from build123d import *

# Parameters (mm, degrees)
BODYSKETCH_R = 0.5969
BODY_DEPTH   = 0.889


with BuildPart() as part:
    # BodySketch → Body (new body)
    with BuildSketch(Plane.XY):
        with BuildLine():
            Line((0.152065789, -5.941654396), (0.22225, -8.683956424))
            ThreePointArc((0.22225, -8.683956424), (1.368573357, -8.578315756), (2.490862191, -8.322024981))
            ThreePointArc((2.490862191, -8.322024981), (2.671680086, -8.204051371), (2.759354342, -8.006754365))
            Line((2.759354342, -8.006754365), (2.871664527, -7.153673811))
            ThreePointArc((2.871664527, -7.153673811), (3.142109784, -6.428451286), (3.702191114, -5.894225443))
            ThreePointArc((3.702191114, -5.894225443), (0, 7.5946), (-3.702191114, -5.894225443))
            ThreePointArc((-3.702191114, -5.894225443), (-3.142109784, -6.428451286), (-2.871664527, -7.153673811))
            Line((-2.871664527, -7.153673811), (-2.759354342, -8.006754365))
            ThreePointArc((-2.759354342, -8.006754365), (-2.671680086, -8.204051371), (-2.490862191, -8.322024981))
            ThreePointArc((-2.490862191, -8.322024981), (-1.368573357, -8.578315756), (-0.22225, -8.683956424))
            Line((-0.22225, -8.683956424), (-0.152065789, -5.941654396))
            ThreePointArc((-0.152065789, -5.941654396), (0, 5.9436), (0.152065789, -5.941654396))
        make_face()
        with Locations((1.0414, -7.445926712)):
            Circle(BODYSKETCH_R, mode=Mode.SUBTRACT)
        with Locations((-1.0414, -7.445926712)):
            Circle(BODYSKETCH_R, mode=Mode.SUBTRACT)
    extrude(amount=BODY_DEPTH)


solid = part.part
For this review, take the finished solid that the model builds, in its own axes (mm). Round coordinates to 2 decimals unless told otherwise and drop trailing zeros. Loops run counter-clockwise (first coordinate to the right, second up) from the corner with the lowest first, then second, coordinate; pieces in that order, holes last. Notation, with made-up numbers: (39, -2.75) - (98, -2.75) arc R30 cw to (98, 31.25) - close; hole circle Ø6 at (-4.5, -16.5). An arc over 180 degrees is marked (long way). One line per question, with ' | ' between items.
Q1. Take a section at B-B (z = 0.4). Give the boundary of the cut face in (x, y), and give its area (3 significant figures).
Taken from the geometry:
outline: (-3.7, -5.89) arc R1.73 cw to (-2.87, -7.15) - (-2.76, -8.01) arc R0.38 ccw to (-2.49, -8.32) arc R8.69 ccw to (-0.22, -8.68) - (-0.15, -5.94) arc R5.94 cw (long way) to (0.15, -5.94) - (0.22, -8.68) arc R8.69 ccw to (2.49, -8.32) arc R0.38 ccw to (2.76, -8.01) - (2.87, -7.15) arc R1.73 cw to (3.7, -5.89) arc R7.25 ccw (long way) to start; hole circle Ø1.19 at (-1.04, -7.45); hole circle Ø1.19 at (1.04, -7.45) | area: 61.5 mm²
Q2. For pin 1 (1 mm diameter, centred on x = -1.04, y = -7.45, fed in from -Z), flat-tipped, find the tip position at first contact; note if it passes through.
Taken from the geometry:
pin 1: passes through
Q3. For line 1 along X through (y, z) = (0.25, 0.75); line 2 along Y through (x, z) = (0, 0.2); line 3 along Y through (x, z) = (5, 0.85), list the stretches that pass through material, from the lowest coordinate up. Write a range as [from, to].
Taken from the geometry:
line 1: x = [-7.25, -5.94], [5.94, 7.25] | line 2: y = [5.94, 7.59] | line 3: y = [-4.91, -3.21], [3.21, 5.6]
Q4. The part is to be moulded in two halves that separate along X. For faces 1 (the cylindrical face through (3.136, -6.438, 0.438)), 2 (the cylindrical face through (-0.259, 5.938, 0.438)), 3 (the cylindrical face through (-3.15, -6.42, 0.44)), say which applies: released by +X, released by -X, zero draft, split by the parting line, or undercut.
Taken from the geometry:
face 1: released by +X | face 2: undercut | face 3: released by -X
Q5. Take a section at A-A (y = 0). Give the boundary of the cut face in (x, z).
Taken from the geometry:
outline: (-7.24, 0) - (-5.94, 0) - (-5.94, 0.89) - (-7.24, 0.89) - close; (5.94, 0) - (7.24, 0) - (7.24, 0.89) - (5.94, 0.89) - close
